Autodesk Inventor part; units mm, degrees
ref_plane "YZ Plane" through (0, 0, 0) normal (1, 0, 0) x (0, 1, 0)
ref_plane "XZ Plane" through (0, 0, 0) normal (0, 1, 0) x (-1, 0, 0)
ref_plane "XY Plane" through (0, 0, 0) normal (0, 0, 1) x (1, 0, 0)
sketch "Эскиз1" plane through (0, 0, 0) normal (0, 0, 1) x (1, 0, 0)
  line L0 (0, 0) -> (-100, 0)
  line L1 (-100, 0) -> (-100, 22.5)
  line L2 (-100, 22.5) -> (0, 22.5)
  line L3 (0, 22.5) -> (0, 0)
  line L4 (-100, 11.25) -> (0, 11.25) construction
  line L5 (0, 11.25) -> (-10.5, 11.25) construction
  circle A0 centre (-10.5, 11.25) radius 10.5 construction
  circle A1 centre (-89, 11.25) radius 10.75
  line L6 (-50, 0) -> (-50, 22.5) construction
  circle A2 centre (-50, 11.25) radius 2
  circle A3 centre (-10.5, 11.25) radius 2
  dimension "d0" = 100
  dimension "d1" = 22.5
  dimension "d2" = 10.5
  dimension "d3" = 11
  dimension "d4" = 21
  dimension "d5" = 21.5
  dimension "d6" = 4
  dimension "d7" = 4
extrude "Выдавливание1" add sketch "Эскиз1" along normal blind 6
sketch "Эскиз2" plane through (0, 0, 0) normal (0, 0, -1) x (-1, 0, 0)
  circle A0 centre (89, 11.25) radius 10.75
  circle A1 centre (89, 11.25) radius 10.75
  point P0 (0, 0)
  point P1 (89.5, 21)
  point P2 (89.5, 0)
  dimension "d23" = 21.5
extrude "Выдавливание2" add sketch "Эскиз2" against normal blind 3
sketch "Эскиз3" plane through (0, 0, 3) normal (0, 0, 1) x (1, 0, 0)
  circle A0 centre (-89, 11.25) radius 10.75
  circle A1 centre (-89, 11.25) radius 2
  point P0 (0, 0)
  point P1 (-89.5, 21)
  point P2 (-89.5, 0)
  dimension "d12" = 4
extrude "Выдавливание3" cut sketch "Эскиз3" against normal blind 3 contours A1
fillet "Сопряжение1" radius 7 4 edges at (0, 22.5, 3) (0, 0, 3) (-100, 22.5, 3) (-100, 0, 3)
sketch "Эскиз4" plane through (0, 0, 0) normal (0, 0, -1) x (-1, 0, 0)
  circle A0 centre (89, 11.25) radius 2
  circle A1 centre (89, 11.25) radius 8 construction
  circle A2 centre (81, 11.25) radius 1
  circle A3 centre (89, 3.25) radius 1
  circle A4 centre (97, 11.25) radius 1
  circle A5 centre (89, 19.25) radius 1
  point P0 (0, 0)
  dimension "d16" = 16
  dimension "d17" = 2
  dimension "d18" = 2
  dimension "d19" = 2
  dimension "d20" = 2
extrude "Выдавливание4" cut sketch "Эскиз4" against normal blind 6 contours A2 | A3 | A4 | A5
properties part number "peregorodka" material "Пластик АБС"
Design review of the part built by this model. Coordinates are the model's own, in mm. A direction names the side the tool comes from. Give positions to 0.01 mm unless a question says otherwise; leave off trailing zeros. Loops run counter-clockwise (first coordinate to the right, second up) from the corner with the lowest first, then second, coordinate; pieces in that order, holes last. Notation, with made-up numbers: M -27.75,-19.5 L 14.25,-19.5 A18 ccw 14.25,5.5 Z; hole C 37.5,82.25 d5. An arc over 180 degrees is marked long. Write item = value, one per line.
Q1. We need section A-A (y = 11.25). Give the boundary of the cut face in (x, z), plus the area to 4 significant figures.
Output values:
outline = M -100,0 L -98,0 L -98,3 L -99.75,3 L -99.75,6 L -100,6 Z; M -96,0 L -91,0 L -91,3 L -96,3 Z; M -87,0 L -82,0 L -82,3 L -87,3 Z; M -80,0 L -52,0 L -52,6 L -78.25,6 L -78.25,3 L -80,3 Z; M -48,0 L -12.5,0 L -12.5,6 L -48,6 Z; M -8.5,0 L 0,0 L 0,6 L -8.5,6 Z
area = 463.5 mm^2
Q2. For faces 5 (the flat face through (-49, 0, 3)), 6 (the flat face through (-89, 9, 3)), list the 3-axis set-ups (+Z, -Z, +X, -X, +Y, -Y) from which the entire face can be reached by the end or side of a thin tool; tool diameter is ignored.
Output values:
face_5 = +Z, -Z, +X, -X, -Y
face_6 = +Z
Q3. Draft analysis for pull direction Y (two halves, no side actions). For faces 1 (the cylindrical face through (-98, 2.1, 3)), 2 (the cylindrical face through (-96, 11.3, 1.5)), 3 (the cylindrical face through (-2, 20.4, 3)), 4 (the cylindrical face through (-11.974, 9.898, 2.958)), state which applies: +Y half, -Y half, draft (parallel to the pull), parting line (faces both ways), or undercut.
Output values:
face_1 = -Y half
face_2 = undercut
face_3 = +Y half
face_4 = undercut
Q4. Insertion check: pin 1 (2.5 mm diameter, centred on x = -89, y = 19.25, fed in from +Z); pin 2 (6 mm diameter, centred on x = -88.5, y = 16.5, fed in from -Z). Each pin has a flat end and moves straight along its axis. Give the tip position at first contact, or say it passes through.
Output values:
pin_1 = 3
pin_2 = 0
Q5. We need section C-C (x = -89). Give the boundary of the cut face in (y, z).
Output values:
outline = M 0,0 L 2.25,0 L 2.25,3 L 0.5,3 L 0.5,6 L 0,6 Z; M 4.25,0 L 9.25,0 L 9.25,3 L 4.25,3 Z; M 13.25,0 L 18.25,0 L 18.25,3 L 13.25,3 Z; M 20.25,0 L 22.5,0 L 22.5,6 L 22,6 L 22,3 L 20.25,3 Z
Q6. To check wall thickness, follow line 1 (X direction, y = 9.5, z = 3.1); line 2 (X direction, y = 10, z = 3.4); line 3 (Y direction, x = -94, z = 4.45). State the ranges of each line that lie inside material, in increasing order. Write a range as [from, to].
Output values:
line_1 = [-100, -99.61], [-78.39, -50.97], [-49.03, -11.47], [-9.53, 0]
line_2 = [-100, -99.68], [-78.32, -51.56], [-48.44, -12.06], [-8.94, 0]
line_3 = [0.07, 1.73], [20.77, 22.43]
Q7. We need section B-B (z = 1.7). Give the boundary of the cut face in (x, y), plus the area to 3 significant figures.
Output values:
outline = M -100,7 A7 ccw -93,0 L -7,0 A7 ccw 0,7 L 0,15.5 A7 ccw -7,22.5 L -93,22.5 A7 ccw -100,15.5 Z; hole C -97,11.25 d2; hole C -89,11.25 d4; hole C -89,3.25 d2; hole C -89,19.25 d2; hole C -81,11.25 d2; hole C -50,11.25 d4; hole C -10.5,11.25 d4
area = 2,160 mm^2
Q8. We need section D-D (y = 6). Give the boundary of the cut face in (x, z).
Output values:
outline = M -99.93,0 L -0.07,0 L -0.07,6 L -79.62,6 L -79.62,3 L -98.38,3 L -98.38,6 L -99.93,6 Z
